from build123d import *

# Parameters (mm, degrees)
BOSS_EXTRUDE2_DEPTH = 11.25
SKETCH3_R           = 1.75
CUT_EXTRUDE1_DEPTH  = 15
SKETCH4_R           = 4.5
CUT_EXTRUDE2_DEPTH  = 5.5
FILLET1_R           = 2
FILLET2_R           = 1
SKETCH5_W           = 43.999736238
SKETCH5_H           = 0.25
CUT_EXTRUDE3_DEPTH  = 20


with BuildPart() as part:
    # Sketch2 → Boss-Extrude2 (new body)
    with BuildSketch(Plane(origin=(0, 0, 0), x_dir=(1, 0, 0), z_dir=(0, 1, 0))):
        with BuildLine():
            Line((4.999419692, -0.076175713), (21.999868119, -0.076175713))
            Line((21.999868119, -0.076175713), (21.999868119, -9.076175713))
            Line((21.999868119, -9.076175713), (8.594942375, -9.076175713))
            ThreePointArc((8.594942375, -9.076175713), (0, -12.5), (-8.594942375, -9.076175713))
            Line((-8.594942375, -9.076175713), (-21.999868119, -9.076175713))
            Line((-21.999868119, -9.076175713), (-21.999868119, -0.076175713))
            Line((-21.999868119, -0.076175713), (-4.999419692, -0.076175713))
            ThreePointArc((-4.999419692, -0.076175713), (0, -5), (4.999419692, -0.076175713))
        make_face()
    extrude(amount=BOSS_EXTRUDE2_DEPTH)

    # Sketch3 → Cut-Extrude1 (cut)
    with BuildSketch(Plane.XY.offset(9.076175713)):
        with Locations((15, 5.625)):
            Circle(SKETCH3_R)
        with Locations((-15, 5.625)):
            Circle(SKETCH3_R)
    extrude(amount=-CUT_EXTRUDE1_DEPTH, mode=Mode.SUBTRACT)

    # Sketch4 → Cut-Extrude2 (cut)
    with BuildSketch(Plane.XY.offset(9.076175713)):
        with Locations((15, 5.625)):
            Circle(SKETCH4_R)
        with Locations((-15, 5.625)):
            Circle(SKETCH4_R)
    extrude(amount=-CUT_EXTRUDE2_DEPTH, mode=Mode.SUBTRACT)

    # Fillet1
    fillet1_edges = [part.edges().sort_by_distance(p)[0] for p in [
        (-21.999868119, 11.25, 4.576175713),
        (21.999868119, 11.25, 4.576175713),
        (21.999868119, 0, 4.576175713),
        (-21.999868119, 0, 4.576175713),
    ]]
    fillet(fillet1_edges, radius=FILLET1_R)

    # Fillet2
    # the kernel refuses this fillet: 1 mm, written as the material it adds along each edge
    with BuildSketch(Plane(origin=(8.594942375, 0, 9.076175713), x_dir=(-0.7363214838652496, 0, 0.6766318588408892), z_dir=(0, 1, 0))) as fillet2_piece_1:
        with BuildLine():
            CenterArc((0.389815045, 0.9998876), FILLET2_R, 227.418998023, 41.721940681)
            Line((-0.286816814, 0.263566116), (0, 0))
            ThreePointArc((0, 0), (0.187411079, 0.001404995), (0.374822159, 0))
        make_face()
    extrude(amount=11.25)
    with BuildSketch(Plane(origin=(-8.594942375, 0, 9.076175713), x_dir=(-1, 0, 0), z_dir=(0, 1, 0))) as fillet2_piece_2:
        with BuildLine():
            CenterArc((0.389526613, 1), FILLET2_R, 228.278059319, 41.721940681)
            ThreePointArc((-0.275989608, 0.253616614), (-0.137044139, 0.127842835), (0, 0))
            Line((0, 0), (0.389526613, 0))
        make_face()
    extrude(amount=11.25)
    # the kernel refuses this fillet: 1 mm, written as the material it takes off along each edge
    with BuildSketch(Plane(origin=(15, 5.625, 9.076175713), x_dir=(1, 0, 0), z_dir=(0, -1, 0))) as fillet2_2_piece_1:
        with BuildLine():
            CenterArc((4.5 + FILLET2_R, -FILLET2_R), FILLET2_R, 90, 90)
            Line((4.5, -FILLET2_R), (4.5, 0))
            Line((4.5, 0), (4.5 + FILLET2_R, 0))
        make_face()
    revolve(axis=Axis((15, 5.625, 9.076175713), (0, 0, 1)), mode=Mode.SUBTRACT)
    with BuildSketch(Plane(origin=(-15, 5.625, 9.076175713), x_dir=(1, 0, 0), z_dir=(0, -1, 0))) as fillet2_2_piece_2:
        with BuildLine():
            CenterArc((4.5 + FILLET2_R, -FILLET2_R), FILLET2_R, 90, 90)
            Line((4.5, -FILLET2_R), (4.5, 0))
            Line((4.5, 0), (4.5 + FILLET2_R, 0))
        make_face()
    revolve(axis=Axis((-15, 5.625, 9.076175713), (0, 0, 1)), mode=Mode.SUBTRACT)
    # the kernel refuses this fillet: 1 mm, written as the material it takes off along each edge
    with BuildSketch(Plane(origin=(0, 11.25, 0), x_dir=(0.6655162213477791, 0, 0.7463833861514965), z_dir=(0.7463833861514965, 0, -0.6655162213477791))) as fillet2_3_piece_1:
        with BuildLine():
            CenterArc((12.5 - FILLET2_R, FILLET2_R), FILLET2_R, 270, 90)
            Line((12.5, FILLET2_R), (12.5, 0))
            Line((12.5, 0), (12.5 - FILLET2_R, 0))
        make_face()
    revolve(axis=Axis((0, 11.25, 0), (0, -1, 0)), revolution_arc=83.443881362, mode=Mode.SUBTRACT)
    with BuildSketch(Plane(origin=(19.999868119, 11.25, 9.076175713), x_dir=(0, 0, -1), z_dir=(-1, 0, 0)), Plane(origin=(-8.984468988, 0, 9.076175713), x_dir=(0, 1, 0), z_dir=(-1, 0, 0))) as fillet2_3_piece_2:
        with BuildLine():
            CenterArc((FILLET2_R, FILLET2_R), FILLET2_R, 180, 90)
            Line((0, FILLET2_R), (0, 0))
            Line((0, 0), (FILLET2_R, 0))
        make_face()
    extrude(amount=11.015399131, mode=Mode.SUBTRACT)
    with BuildSketch(Plane(origin=(21.999868119, 2, 9.076175713), x_dir=(-1, 0, 0), z_dir=(0, 1, 0))) as fillet2_3_piece_3:
        with BuildLine():
            CenterArc((FILLET2_R, -FILLET2_R), FILLET2_R, 90, 90)
            Line((0, -FILLET2_R), (0, 0))
            Line((0, 0), (FILLET2_R, 0))
        make_face()
    extrude(amount=7.25, mode=Mode.SUBTRACT)
    with BuildSketch(Plane(origin=(19.999868119, 9.25, 9.076175713), x_dir=(0, 1, 0), z_dir=(-1, 0, 0))) as fillet2_3_piece_4:
        with BuildLine():
            CenterArc((2 - FILLET2_R, FILLET2_R), FILLET2_R, 270, 90)
            Line((2, FILLET2_R), (2, 0))
            Line((2, 0), (2 - FILLET2_R, 0))
        make_face()
    revolve(axis=Axis((19.999868119, 9.25, 9.076175713), (0, 0, -1)), revolution_arc=90, mode=Mode.SUBTRACT)
    with BuildSketch(Plane(origin=(19.999868119, 2, 9.076175713), x_dir=(0, -1, 0), z_dir=(-1, 0, 0))) as fillet2_3_piece_5:
        with BuildLine():
            CenterArc((2 - FILLET2_R, -FILLET2_R), FILLET2_R, 0, 90)
            Line((2 - FILLET2_R, 0), (2, 0))
            Line((2, 0), (2, -FILLET2_R))
        make_face()
    revolve(axis=Axis((19.999868119, 2, 9.076175713), (0, 0, 1)), revolution_arc=90, mode=Mode.SUBTRACT)
    with BuildSketch(Plane(origin=(-8.984468988, 11.25, 9.076175713), x_dir=(0, -1, 0), z_dir=(-1, 0, 0)), Plane(origin=(19.999868119, 0, 9.076175713), x_dir=(0, 0, -1), z_dir=(-1, 0, 0))) as fillet2_3_piece_6:
        with BuildLine():
            CenterArc((FILLET2_R, -FILLET2_R), FILLET2_R, 90, 90)
            Line((0, -FILLET2_R), (0, 0))
            Line((0, 0), (FILLET2_R, 0))
        make_face()
    extrude(amount=11.015399131, mode=Mode.SUBTRACT)
    with BuildSketch(Plane(origin=(-21.999868119, 2, 9.076175713), x_dir=(1, 0, 0), z_dir=(0, 1, 0))) as fillet2_3_piece_7:
        with BuildLine():
            CenterArc((FILLET2_R, FILLET2_R), FILLET2_R, 180, 90)
            Line((0, FILLET2_R), (0, 0))
            Line((0, 0), (FILLET2_R, 0))
        make_face()
    extrude(amount=7.25, mode=Mode.SUBTRACT)
    with BuildSketch(Plane(origin=(-19.999868119, 9.25, 9.076175713), x_dir=(0, 1, 0), z_dir=(1, 0, 0))) as fillet2_3_piece_8:
        with BuildLine():
            CenterArc((2 - FILLET2_R, -FILLET2_R), FILLET2_R, 360, 90)
            Line((2, -FILLET2_R), (2, 0))
            Line((2, 0), (2 - FILLET2_R, 0))
        make_face()
    revolve(axis=Axis((-19.999868119, 9.25, 9.076175713), (0, 0, 1)), revolution_arc=90, mode=Mode.SUBTRACT)
    with BuildSketch(Plane(origin=(-19.999868119, 2, 9.076175713), x_dir=(0, -1, 0), z_dir=(1, 0, 0))) as fillet2_3_piece_9:
        with BuildLine():
            CenterArc((2 - FILLET2_R, FILLET2_R), FILLET2_R, 270, 90)
            Line((2, FILLET2_R), (2, 0))
            Line((2, 0), (2 - FILLET2_R, 0))
        make_face()
    revolve(axis=Axis((-19.999868119, 2, 9.076175713), (0, 0, -1)), revolution_arc=90, mode=Mode.SUBTRACT)
    with BuildSketch(Plane(origin=(0, 0, 0), x_dir=(0.6655162213477791, 0, 0.7463833861514965), z_dir=(0.7463833861514965, 0, -0.6655162213477791))) as fillet2_3_piece_10:
        with BuildLine():
            CenterArc((12.5 - FILLET2_R, -FILLET2_R), FILLET2_R, 0, 90)
            Line((12.5, -FILLET2_R), (12.5, 0))
            Line((12.5, 0), (12.5 - FILLET2_R, 0))
        make_face()
    revolve(axis=Axis((0, 0, 0), (0, -1, 0)), revolution_arc=83.443881362, mode=Mode.SUBTRACT)
    with BuildSketch(Plane(origin=(8.984468988, 0, 10.076175713), x_dir=(-0.6655162213477794, 0, -0.7463833861514964), z_dir=(-0.7463833861514964, 0, 0.6655162213477794))) as fillet2_3_piece_11:
        with BuildLine():
            CenterArc((1 + FILLET2_R, -FILLET2_R), FILLET2_R, 90, 90)
            Line((1, -FILLET2_R), (1, 0))
            Line((1, 0), (1 + FILLET2_R, 0))
        make_face()
    revolve(axis=Axis((8.984468988, 0, 10.076175713), (0, -1, 0)), revolution_arc=41.721940681, mode=Mode.SUBTRACT)
    with BuildSketch(Plane(origin=(-8.984468988, 0, 10.076175713), x_dir=(0, 0, -1), z_dir=(-1, 0, 0))) as fillet2_3_piece_12:
        with BuildLine():
            CenterArc((1 + FILLET2_R, -FILLET2_R), FILLET2_R, 90, 90)
            Line((1, -FILLET2_R), (1, 0))
            Line((1, 0), (1 + FILLET2_R, 0))
        make_face()
    revolve(axis=Axis((-8.984468988, 0, 10.076175713), (0, -1, 0)), revolution_arc=41.721940681, mode=Mode.SUBTRACT)
    with BuildSketch(Plane(origin=(-8.984468988, 11.25, 10.076175713), x_dir=(0, 0, -1), z_dir=(-1, 0, 0))) as fillet2_3_piece_13:
        with BuildLine():
            CenterArc((1 + FILLET2_R, FILLET2_R), FILLET2_R, 180, 90)
            Line((1 + FILLET2_R, 0), (1, 0))
            Line((1, 0), (1, FILLET2_R))
        make_face()
    revolve(axis=Axis((-8.984468988, 11.25, 10.076175713), (0, -1, 0)), revolution_arc=41.721940681, mode=Mode.SUBTRACT)
    with BuildSketch(Plane(origin=(8.984468988, 11.25, 10.076175713), x_dir=(-0.6655162213477794, 0, -0.7463833861514964), z_dir=(-0.7463833861514964, 0, 0.6655162213477794))) as fillet2_3_piece_14:
        with BuildLine():
            CenterArc((1 + FILLET2_R, FILLET2_R), FILLET2_R, 180, 90)
            Line((1, FILLET2_R), (1, 0))
            Line((1, 0), (1 + FILLET2_R, 0))
        make_face()
    revolve(axis=Axis((8.984468988, 11.25, 10.076175713), (0, -1, 0)), revolution_arc=41.721940681, mode=Mode.SUBTRACT)

    # Sketch5 → Cut-Extrude3 (cut)
    with BuildSketch(Plane(origin=(0, 11.25, 0), x_dir=(1, 0, 0), z_dir=(0, 1, 0))):
        with Locations((0, -0.201175713)):
            Rectangle(SKETCH5_W, SKETCH5_H)
    extrude(amount=-CUT_EXTRUDE3_DEPTH, mode=Mode.SUBTRACT)


solid = part.part
Model file for the job. Use its own axes, mm. A direction names the side the tool comes from. Give positions to 0.01 mm unless a question says otherwise; leave off trailing zeros. Loops run counter-clockwise (first coordinate to the right, second up) from the corner with the lowest first, then second, coordinate; pieces in that order, holes last.
1) Wall check: line 1 (Y direction, x = -15, z = 6.7) (3 decimals); line 2 (X direction, y = 4.25, z = 2.5); line 3 (X direction, y = 8, z = 7.5). Give the ranges that are in metal, low to high.
2) Saw through at A-A (z = 3). Write the cut outline in (x, y) (3 decimals).
3) Flat gauge pins, fed straight in: pin 1 Ø1.5 at (x, y) = (7, 7) entering from +Z; pin 2 Ø3.5 at (x, y) = (-19, 4) entering from +Z; pin 3 Ø4.5 at (x, y) = (13, 7) entering from +Z; pin 4 Ø5.5 at (x, y) = (-15, 5.625) entering from -Z. Where does each tip first touch, or does it go through?
4) Pull direction X, two halves, no side cores. Call faces 6 (the flat face through (13, 7, 0.326)), 7 (the cylindrical face through (0.1, 5.6, 12.5)), 8 (the cylindrical face through (-18.571, 2.887, 5.858)): +X half, -X half, draft (parallel to the pull), parting line (faces both ways), or undercut.
5) Saw through at C-C (x = 0). Write the cut outline in (y, z).
6) Saw through at D-D (y = 5). Count the separate pieces of the cut face and the enclosed holes in it, plus the area to 3 significant figures.
7) Tool access for faces 1 (the flat face through (-13, 6, 3.576)), 2 (the flat face through (-13.6, 7, 0.326)), 3 (the cylindrical face through (14.57, 10.95, 8.79)), 4 (the cylindrical face through (-14.42, 10.95, 8.79)), 5 (the cylindrical face through (14.57, 0.29, 8.78)): list every direction of +Z, -Z, +X, -X, +Y, -Y with a clear straight run to the whole face (end or side of a thin tool).
Answer block:
1. line 1: y = 0 to 1.125, 10.125 to 11.25
1. line 2: x = -22 to -16.08, -13.92 to -4.33, 4.33 to 13.92, 16.08 to 22
1. line 3: x = -22 to -18.82, -11.18 to 11.18, 18.82 to 22
2. outline: (-22, 2) arc R2 ccw to (-20, 0) - (-4, 0) - (-4, 11.25) - (-20, 11.25) arc R2 ccw to (-22, 9.25) - close; (4, 0) - (20, 0) arc R2 ccw to (22, 2) - (22, 9.25) arc R2 ccw to (20, 11.25) - (4, 11.25) - close; hole circle Ø3.5 at (-15, 5.625); hole circle Ø3.5 at (15, 5.625)
3. pin 1: stops at z = 10.83
3. pin 2: stops at z = 9.08
3. pin 3: stops at z = 8.64
3. pin 4: stops at z = 0.33
4. face 6: draft
4. face 7: parting line
4. face 8: undercut
5. outline: (0, 5) - (11.25, 5) - (11.25, 11.5) arc R1 ccw to (10.25, 12.5) - (1, 12.5) arc R1 ccw to (0, 11.5) - close
6. separate pieces: 3
6. enclosed holes: 0
6. area: 269 mm2
7. face 1: +Z
7. face 2: -Z, +X, -X, +Y, -Y
7. face 3: +Z, +X, +Y
7. face 4: +Z, -X, +Y
7. face 5: +Z, +X, -Y
